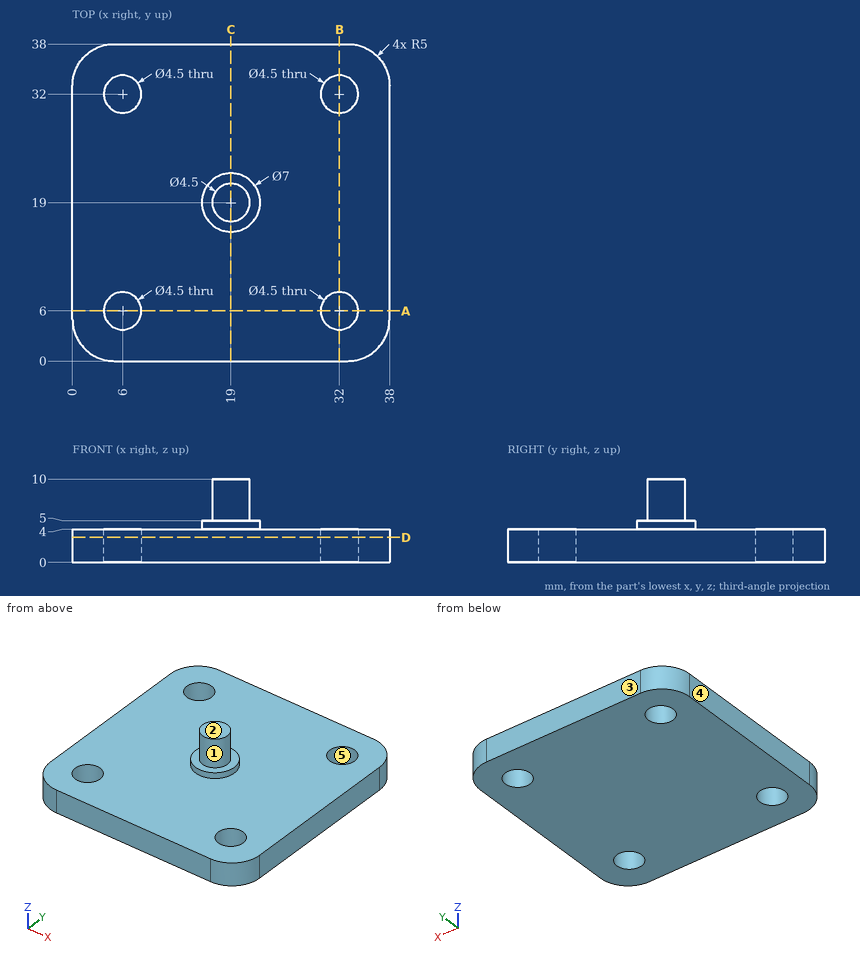
Here's the drawing with two shaded views (mm, measured from the low corner). I have some questions. A direction names the side the tool comes from. Coordinates: 2 decimals unless noted, no trailing zeros. Order: outer loops, then holes, each group sorted by start corner. A loop starts at its lowest first (then second) coordinate and runs counter-clockwise, first axis right, second up. Notation, with made-up numbers: (61, -17.5) - (96, -17.5) arc R21 ccw to (96, 15.5) - close; hole circle Ø2 at (-37, 60.25). An arc over 180 degrees is marked (long way). Use CSV: the item, a comma, the result in double quotes. Start each with the question number.
1. Suppose I cut it at C-C on x = 19. List the corners of the cut face in (y, z) for me, then the cut area to 4 significant figures.
2. For the marked faces 1 and 2, which set-ups out of +Z, -Z, +X, -X, +Y, -Y let a thin tool reach every point of the face, with its end or its side?
3. If we mould it in two halves opening along X, with no side actions, what happens to the marked faces 3, 4 and 5? For each: +X half, -X half, draft (parallel to the pull), parting line (faces both ways), or undercut.
4. Suppose I cut it at A-A on y = 6. List the corners of the cut face in (x, z) for me, then the cut area to 3 significant figures.
5. Suppose I cut it at D-D on z = 3. List the corners of the cut face in (x, y) for me.
6. Please list where these lines run through material, in increasing order: line 1 (Y direction, x = 6, z = 3.05); line 2 (Y direction, x = 7, z = 1); line 3 (Z direction, x = 14.5, y = 33). Write a range as from..to.
7. I'm going to push flat-ended pins straight in: pin 1 (2.5 mm diameter, centred on x = 32, y = 6, fed in from -Z); pin 2 (5 mm diameter, centred on x = 32, y = 32, fed in from +Z). Where does each tip first touch, or does it pass through?
Output:
1,outline,"(0, 0) - (38, 0) - (38, 4) - (22.5, 4) - (22.5, 5) - (21.25, 5) - (21.25, 10) - (16.75, 10) - (16.75, 5) - (15.5, 5) - (15.5, 4) - (0, 4) - close"
1,area,"181.5 mm2"
2,face 1,"+Z"
2,face 2,"+Z, +X, -X, +Y, -Y"
3,face 3,"draft"
3,face 4,"-X half"
3,face 5,"undercut"
4,outline,"(0, 0) - (3.75, 0) - (3.75, 4) - (0, 4) - close; (8.25, 0) - (29.75, 0) - (29.75, 4) - (8.25, 4) - close; (34.25, 0) - (38, 0) - (38, 4) - (34.25, 4) - close"
4,area,"116 mm2"
5,outline,"(0, 5) arc R5 ccw to (5, 0) - (33, 0) arc R5 ccw to (38, 5) - (38, 33) arc R5 ccw to (33, 38) - (5, 38) arc R5 ccw to (0, 33) - close; hole circle Ø4.5 at (6, 6); hole circle Ø4.5 at (6, 32); hole circle Ø4.5 at (32, 6); hole circle Ø4.5 at (32, 32)"
6,line 1,"y = 0..3.75, 8.25..29.75, 34.25..38"
6,line 2,"y = 0..3.98, 8.02..29.98, 34.02..38"
6,line 3,"z = 0..4"
7,pin 1,"passes through"
7,pin 2,"stops at z = 4"
